Can you work these out from the model? Positions are in its coordinate system, mm. A direction names the side the tool comes from. Give positions to 0.01 mm unless a question says otherwise; leave off trailing zeros. Write each loop counter-clockwise with the first axis right and the second up, starting at its lowest first coordinate (ties: lowest second). Pieces come first, ordered by that corner, then holes. Notation, with made-up numbers: (44, 18.5) -> (85, 18.5) arc R26 ccw to (85, 43.5) -> close; hole circle Ø3 at (-38, -13.5). An arc over 180 degrees is marked (long way). One line per item, written item: value.
from build123d import *

# Parameters (mm, degrees)
EXTRUDE_1_DEPTH     = 5
SKETCH_2_R          = 1.5
SKETCH_2_R_2        = 4
CUT_EXTRUDE_1_DEPTH = 5
SKETCH_3_W          = 3
SKETCH_3_H          = 4
CUT_EXTRUDE_2_DEPTH = 5
SKETCH_4_R          = 4
SKETCH_4_R_2        = 1.1
SKETCH_4_W          = 3
SKETCH_4_H          = 4
CUT_EXTRUDE_4_DEPTH = 10
SKETCH_5_W          = 50
SKETCH_5_H          = 20
CUT_EXTRUDE_5_DEPTH = 10
SKETCH_6_W          = 15
SKETCH_6_H          = 20
EXTRUDE_2_DEPTH     = 7.7
SKETCH_7_R          = 2.25
CUT_EXTRUDE_6_DEPTH = 20
SKETCH_8_W          = 15
SKETCH_8_H          = 10
SKETCH_8_R          = 2
EXTRUDE_3_DEPTH     = 12.7
SKETCH_9_W          = 3.2
SKETCH_9_H          = 20
CUT_EXTRUDE_7_DEPTH = 8


with BuildPart() as part:
    # 草图1 → 凸台-拉伸1 (new body)
    with BuildSketch(Plane(origin=(0, 0, 0), x_dir=(1, 0, 0), z_dir=(0, 1, 0))):
        with BuildLine():
            Line((-41.199983302, 20), (78.800016698, 20))
            Line((78.800016698, 20), (78.800016698, 0))
            Line((78.800016698, 0), (-41.199983302, 0))
            ThreePointArc((-41.199983302, 0), (-51.199983302, 10), (-41.199983302, 20))
        make_face()
    extrude(amount=EXTRUDE_1_DEPTH)

    # 草图2 → 切除-拉伸1 (cut)
    with BuildSketch(Plane(origin=(0, 5, 0), x_dir=(1, 0, 0), z_dir=(0, 1, 0))):
        with Locations(Location((-48.199983302, 10, 0), (0, 0, 270))):
            Circle(SKETCH_2_R)
        with BuildLine():
            ThreePointArc((-39.699983302, 17), (-40.13932313, 18.060660172), (-41.199983302, 18.5))
            Line((-41.199983302, 18.5), (-41.199983302, 17))
            Line((-41.199983302, 17), (-41.199983302, 15.5))
            ThreePointArc((-41.199983302, 15.5), (-40.13932313, 15.939339828), (-39.699983302, 17))
        make_face()
        with BuildLine():
            Line((-41.199983302, 17), (-41.199983302, 18.5))
            ThreePointArc((-41.199983302, 18.5), (-42.699983302, 17), (-41.199983302, 15.5))
            Line((-41.199983302, 15.5), (-41.199983302, 17))
        make_face()
        with Locations(Location((-34.199983302, 10, 0), (0, 0, 270))):
            Circle(SKETCH_2_R)
        with BuildLine():
            ThreePointArc((-39.699983302, 3), (-40.13932313, 4.060660172), (-41.199983302, 4.5))
            Line((-41.199983302, 4.5), (-41.199983302, 3))
            Line((-41.199983302, 3), (-41.199983302, 1.5))
            ThreePointArc((-41.199983302, 1.5), (-40.13932313, 1.939339828), (-39.699983302, 3))
        make_face()
        with BuildLine():
            Line((-41.199983302, 3), (-41.199983302, 4.5))
            ThreePointArc((-41.199983302, 4.5), (-42.699983302, 3), (-41.199983302, 1.5))
            Line((-41.199983302, 1.5), (-41.199983302, 3))
        make_face()
        with Locations(Location((-41.199983302, 10, 0), (0, 0, 270))):
            Circle(SKETCH_2_R_2)
    extrude(amount=-CUT_EXTRUDE_1_DEPTH, mode=Mode.SUBTRACT)

    # 草图3 → 切除-拉伸2 (cut)
    with BuildSketch(Plane(origin=(0, 5, 0), x_dir=(1, 0, 0), z_dir=(0, 1, 0))):
        with Locations((-12.699983302, 14)):
            Rectangle(SKETCH_3_W, SKETCH_3_H)
        with Locations((-12.699983302, 6)):
            Rectangle(SKETCH_3_W, SKETCH_3_H)
    extrude(amount=-CUT_EXTRUDE_2_DEPTH, mode=Mode.SUBTRACT)

    # 草图4 → 切除-拉伸4 (cut)
    with BuildSketch(Plane(origin=(0, 5, 0), x_dir=(1, 0, 0), z_dir=(0, 1, 0))):
        with Locations(Location((69.300016698, 10, 0), (0, 0, 270))):
            Circle(SKETCH_4_R)
        with Locations(Location((76.7246379, 17.424621202, 0), (0, 0, 270))):
            Circle(SKETCH_4_R_2)
        with Locations(Location((62.300016698, 10, 0), (0, 0, 270))):
            Circle(SKETCH_4_R_2)
        with Locations((50.800016698, 6)):
            Rectangle(SKETCH_4_W, SKETCH_4_H)
        with Locations((50.800016698, 14)):
            Rectangle(SKETCH_4_W, SKETCH_4_H)
        with Locations(Location((76.7246379, 2.575378798, 0), (0, 0, 270))):
            Circle(SKETCH_4_R_2)
        with Locations(Location((61.875395496, 2.575378798, 0), (0, 0, 270))):
            Circle(SKETCH_4_R_2)
        with Locations(Location((61.875395496, 17.424621202, 0), (0, 0, 270))):
            Circle(SKETCH_4_R_2)
        with Locations(Location((69.300016698, 17, 0), (0, 0, 270))):
            Circle(SKETCH_4_R_2)
        with Locations(Location((76.300016698, 10, 0), (0, 0, 270))):
            Circle(SKETCH_4_R_2)
        with Locations(Location((69.300016698, 3, 0), (0, 0, 270))):
            Circle(SKETCH_4_R_2)
    extrude(amount=-CUT_EXTRUDE_4_DEPTH, mode=Mode.SUBTRACT)

    # 草图5 → 切除-拉伸5 (cut)
    with BuildSketch(Plane(origin=(0, 5, 0), x_dir=(1, 0, 0), z_dir=(0, 1, 0))):
        with Locations((53.800016698, 10)):
            Rectangle(SKETCH_5_W, SKETCH_5_H)
    extrude(amount=-CUT_EXTRUDE_5_DEPTH, mode=Mode.SUBTRACT)

    # 草图6 → 凸台-拉伸2 (add)
    with BuildSketch(Plane(origin=(0, 5, 0), x_dir=(1, 0, 0), z_dir=(0, 1, 0))):
        with Locations((21.300016698, 10)):
            Rectangle(SKETCH_6_W, SKETCH_6_H)
    extrude(amount=EXTRUDE_2_DEPTH)

    # 草图7 → 切除-拉伸6 (cut)
    with BuildSketch(Plane(origin=(28.800016698, 0, 0), x_dir=(0, 0, -1), z_dir=(1, 0, 0))):
        with Locations((5, 8.8)):
            Circle(SKETCH_7_R)
        with Locations((15, 8.8)):
            Circle(SKETCH_7_R)
    extrude(amount=-CUT_EXTRUDE_6_DEPTH, mode=Mode.SUBTRACT)

    # 草图8 → 凸台-拉伸3 (add)
    # profile 1 of 2: a face of its own
    with BuildSketch(Plane(origin=(0, 12.7, 0), x_dir=(1, 0, 0), z_dir=(0, 1, 0))):
        with Locations((21.300016698, 25)):
            Rectangle(SKETCH_8_W, SKETCH_8_H)
        with Locations(Location((21.300016698, 25, 0), (0, 0, 270))):
            Circle(SKETCH_8_R, mode=Mode.SUBTRACT)
    # profile 2 of 2: a face of its own
    with BuildSketch(Plane(origin=(0, 12.7, 0), x_dir=(1, 0, 0), z_dir=(0, 1, 0))):
        with Locations((21.300016698, -5)):
            Rectangle(SKETCH_8_W, SKETCH_8_H)
        with Locations(Location((21.300016698, -5, 0), (0, 0, 270))):
            Circle(SKETCH_8_R, mode=Mode.SUBTRACT)
    extrude(amount=-EXTRUDE_3_DEPTH)

    # 草图9 → 切除-拉伸7 (cut)
    with BuildSketch(Plane(origin=(0, 12.7, 0), x_dir=(1, 0, 0), z_dir=(0, 1, 0))):
        with Locations((21.300016698, 10)):
            Rectangle(SKETCH_9_W, SKETCH_9_H)
    extrude(amount=-CUT_EXTRUDE_7_DEPTH, mode=Mode.SUBTRACT)


solid = part.part
1) We'd pull the mould along Z, two halves only. Please class faces 4 (the face through (-18, 5, -10)), 5 (the face through (-13, 3, -12)), 6 (the face through (21, 6, -30)), 7 (the face through (16.791, 9.476, -17.146)): released by +Z, released by -Z, zero draft, split by the parting line, or undercut.
Answer list:
face 4: zero draft
face 5: undercut
face 6: released by -Z
face 7: undercut
2) I need wall thicknesses on L1, parallel to X at y = 1.35, z = -10; L2, parallel to Y at x = 18.25, z = -5; L3, parallel to X at y = 7.5, z = -8. Which ranges of each line are inside material? Lowest first, please.
Answer list:
L1: x = -51.2 to -49.7, -46.7 to -45.2, -37.2 to -35.7, -32.7 to 28.8
L2: y = 0 to 6.55, 11.05 to 12.7
L3: x = 13.8 to 19.7, 22.9 to 28.8
3) If we section it at B-B (z = 5): Write out the boundary of the cut face in (x, y).
Answer list:
outline: (13.8, 0) -> (19.3, 0) -> (19.3, 12.7) -> (13.8, 12.7) -> close; (23.3, 0) -> (28.8, 0) -> (28.8, 12.7) -> (23.3, 12.7) -> close
4) If we section it at D-D (x = 6): Write out the boundary of the cut face in (y, z).
Answer list:
outline: (0, -20) -> (5, -20) -> (5, 0) -> (0, 0) -> close
5) Will these pins go through, and if not, where does the flat tip stop? pin 1 (16 mm diameter, centred on x = -28, z = -5, fed in from +Y); pin 2 (1.8 mm diameter, centred on x = -34.2, z = -10, fed in from +Y); pin 3 (1 mm diameter, centred on y = 5, z = -1.5, fed in from -X); pin 4 (3 mm diameter, centred on y = 6, z = 2.5, fed in from -X).
Answer list:
pin 1: stops at y = 5
pin 2: passes through
pin 3: stops at x = -47.2
pin 4: stops at x = 13.8
6) If we section it at A-A (y = 10): Write out the boundary of the cut face in (x, z).
Answer list:
outline: (13.8, -30) -> (28.8, -30) -> (28.8, -16.9) -> (22.9, -16.9) -> (22.9, -20) -> (19.7, -20) -> (19.7, -16.9) -> (13.8, -16.9) -> close; (13.8, -13.1) -> (19.7, -13.1) -> (19.7, -6.9) -> (13.8, -6.9) -> close; (13.8, -3.1) -> (19.7, -3.1) -> (19.7, 0) -> (22.9, 0) -> (22.9, -3.1) -> (28.8, -3.1) -> (28.8, 10) -> (13.8, 10) -> close; (22.9, -13.1) -> (28.8, -13.1) -> (28.8, -6.9) -> (22.9, -6.9) -> close; hole circle Ø4 at (21.3, -25); hole circle Ø4 at (21.3, 5)
7) For faces 1 (the face through (25.891, 10.697, -6.21)), 2 (the face through (-13, 3, -4)), 3 (the face through (19.7, 9, -10)), which set-ups out of +Z, -Z, +X, -X, +Y, -Y let a thin tool reach every point of the face, with its end or its side?
Answer list:
face 1: +X, -X
face 2: +Y, -Y
face 3: +Y
8) If we section it at C-C (y = 1.5): State how many separate pieces and enclosed holes the cut face has, and give its area (3 significant figures).
Answer list:
separate pieces: 1
enclosed holes: 9
area: 1,730 mm^2
